from build123d import *

# Parameters (mm, degrees)
BOSS_EXTRUDE1_DEPTH = 3
SKETCH3_R           = 1.6
CUT_EXTRUDE1_DEPTH  = 3
SKETCH4_W           = 3
SKETCH4_H           = 10
SKETCH4_W_2         = 10
SKETCH4_H_2         = 3
CUT_EXTRUDE2_DEPTH  = 3
SKETCH5_R           = 2
BOSS_EXTRUDE2_DEPTH = 3
FILLET1_R           = 3


with BuildPart() as part:
    # Sketch1 → Boss-Extrude1 (new body)
    with BuildSketch(Plane.XY):
        with BuildLine():
            Line((52, -24), (52, 42.5))
            ThreePointArc((52, 42.5), (50.535533906, 46.035533906), (47, 47.5))
            Line((47, 47.5), (-21, 47.5))
            ThreePointArc((-21, 47.5), (-24.535533906, 46.035533906), (-26, 42.5))
            Line((-26, 42.5), (-26, -24))
            ThreePointArc((-26, -24), (-24.535533906, -27.535533906), (-21, -29))
            Line((-21, -29), (47, -29))
            ThreePointArc((47, -29), (50.535533906, -27.535533906), (52, -24))
        make_face()
    extrude(amount=BOSS_EXTRUDE1_DEPTH)

    # Sketch3 → Cut-Extrude1 (cut)
    with BuildSketch(Plane(origin=(0, 0, 0), x_dir=(-1, 0, 0), z_dir=(0, 0, -1))):
        with Locations((17.5, 40)):
            Circle(SKETCH3_R)
        with Locations((-45.5, 19.5)):
            Circle(SKETCH3_R)
    extrude(amount=-CUT_EXTRUDE1_DEPTH, mode=Mode.SUBTRACT)

    # Sketch4 → Cut-Extrude2 (cut)
    with BuildSketch(Plane(origin=(0, 0, 0), x_dir=(-1, 0, 0), z_dir=(0, 0, -1))):
        with Locations((24.5, 24.25)):
            Rectangle(SKETCH4_W, SKETCH4_H)
        with Locations((24.5, -5.75)):
            Rectangle(SKETCH4_W, SKETCH4_H)
        with Locations((-50.5, -5.75)):
            Rectangle(SKETCH4_W, SKETCH4_H)
        with Locations((-50.5, 24.25)):
            Rectangle(SKETCH4_W, SKETCH4_H)
        with Locations((2, 46)):
            Rectangle(SKETCH4_W_2, SKETCH4_H_2)
        with Locations((-28, 46)):
            Rectangle(SKETCH4_W_2, SKETCH4_H_2)
        with Locations((-28, -27.5)):
            Rectangle(SKETCH4_W_2, SKETCH4_H_2)
        with Locations((2, -27.5)):
            Rectangle(SKETCH4_W_2, SKETCH4_H_2)
    extrude(amount=-CUT_EXTRUDE2_DEPTH, mode=Mode.SUBTRACT)

    # Sketch5 → Boss-Extrude2 (add)
    # profile 1 of 4: a face of its own
    with BuildSketch(Plane.XY.offset(3)):
        with BuildLine():
            Line((-18, 47.5), (-10, 47.5))
            Line((-10, 47.5), (-10, 50.5))
            ThreePointArc((-10, 50.5), (-14, 54.5), (-18, 50.5))
            Line((-18, 50.5), (-18, 47.5))
        make_face()
        with Locations((-14, 50.5)):
            Circle(SKETCH5_R, mode=Mode.SUBTRACT)
    # profile 2 of 4: a face of its own
    with BuildSketch(Plane.XY.offset(3)):
        with BuildLine():
            Line((36, 47.5), (36, 50.5))
            ThreePointArc((36, 50.5), (40, 54.5), (44, 50.5))
            Line((44, 50.5), (44, 47.5))
            Line((44, 47.5), (36, 47.5))
        make_face()
        with Locations(Location((40, 50.5, 0), (0, 0, 180))):
            Circle(SKETCH5_R, mode=Mode.SUBTRACT)
    # profile 3 of 4: a face of its own
    with BuildSketch(Plane.XY.offset(3)):
        with BuildLine():
            Line((44, -29), (36, -29))
            Line((36, -29), (36, -32))
            ThreePointArc((36, -32), (40, -36), (44, -32))
            Line((44, -32), (44, -29))
        make_face()
        with Locations((40, -32)):
            Circle(SKETCH5_R, mode=Mode.SUBTRACT)
    # profile 4 of 4: a face of its own
    with BuildSketch(Plane.XY.offset(3)):
        with BuildLine():
            Line((-10, -29), (-10, -32))
            ThreePointArc((-10, -32), (-14, -36), (-18, -32))
            Line((-18, -32), (-18, -29))
            Line((-18, -29), (-10, -29))
        make_face()
        with Locations(Location((-14, -32, 0), (0, 0, 180))):
            Circle(SKETCH5_R, mode=Mode.SUBTRACT)
    extrude(amount=-BOSS_EXTRUDE2_DEPTH)

    # Fillet1
    fillet1_edges = [part.edges().sort_by_distance(p)[0] for p in [
        (-10, 47.5, 1.5),
        (-18, 47.5, 1.5),
        (36, 47.5, 1.5),
        (44, 47.5, 1.5),
        (44, -29, 1.5),
        (36, -29, 1.5),
        (-10, -29, 1.5),
        (-18, -29, 1.5),
    ]]
    fillet(fillet1_edges, radius=FILLET1_R - 0.0001)  # a hair under: the kernel refuses the full size


solid = part.part
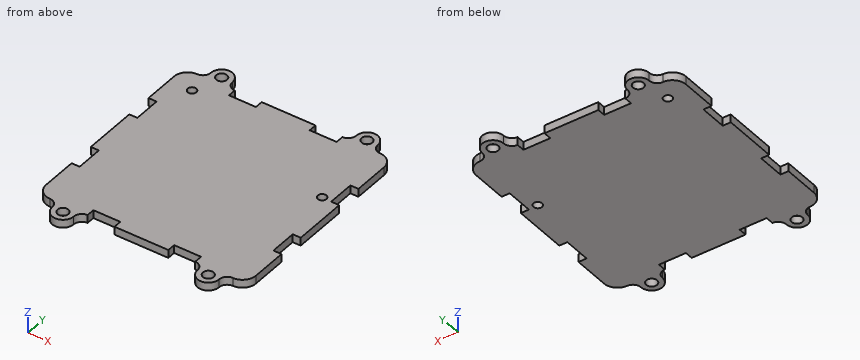
Part model, mm, in its own coordinate system. Round coordinates to 2 decimals unless told otherwise and drop trailing zeros. Write each loop counter-clockwise with the first axis right and the second up, starting at its lowest first coordinate (ties: lowest second). Pieces come first, ordered by that corner, then holes. Notation, with made-up numbers: M 22,61 L 40,61 A15 cw 40,73 Z; hole C 59,56.25 d11. An arc over 180 degrees is marked long. Return JSON: item names as keys, results as strings. Group by question number.
(1) Saw through at D-D on y = 25.5. Write the cut outline in (x, z), then the cut area to 3 significant figures.
(2) Saw through at A-A on y = 40. Write the cut outline in (x, z), then the cut area to 3 significant figures.
(3) Saw through at C-C on z = 1.8. Count the separate pieces of the cut face and the enclosed holes in it, then the cut area to 3 significant figures.
(4) Pin check, flat tips, straight feed: pin 1 Ø0.9 at (x, z) = (16.5, 2) entering from -Y; pin 2 Ø0.9 at (y, z) = (46, 1) entering from +X; pin 3 Ø0.9 at (x, z) = (26, 1) entering from +Y. Stop position of each tip, or through.
(5) Drill centre lines: probe 1 along Y at (x, z) = (40, 1.45); probe 2 along X at (y, z) = (51.5, 0.8); probe 3 along Y at (x, z) = (-12.5, 2.25). Where is each one in solid material? Low to high.
(6) Saw through at B-B on x = 40. Write the cut outline in (y, z).
Returned:
{
 "1": {"outline": "M -23,0 L 49,0 L 49,3 L -23,3 Z", "area": "216 mm²"},
 "2": {"outline": "M -26,0 L -19.1,0 L -19.1,3 L -26,3 Z; M -15.9,0 L 52,0 L 52,3 L -15.9,3 Z", "area": "224 mm²"},
 "3": {"separate pieces": "1", "enclosed holes": "6", "area": "5,850 mm²"},
 "4": {"pin 1": "y = -29", "pin 2": "x = 50.96", "pin 3": "y = 44.5"},
 "5": {"probe 1": "-36 to -34, -30 to 48.5, 52.5 to 54.5", "probe 2": "-17.87 to -15.73, -12.27 to -10.13, 36.13 to 38.27, 41.73 to 43.87", "probe 3": "-35.71 to -33.32, -30.68 to 49.18, 51.82 to 54.21"},
 "6": {"outline": "M -36,0 L -34,0 L -34,3 L -36,3 Z; M -30,0 L 48.5,0 L 48.5,3 L -30,3 Z; M 52.5,0 L 54.5,0 L 54.5,3 L 52.5,3 Z"}
}
